Could you check a few things on this model? Use its own coordinates, in mm. Face numbers are marked on the shaded views. A direction names the side the tool comes from. Coordinates: 2 decimals unless noted, no trailing zeros. Loops run counter-clockwise (first coordinate to the right, second up) from the corner with the lowest first, then second, coordinate; pieces in that order, holes last.
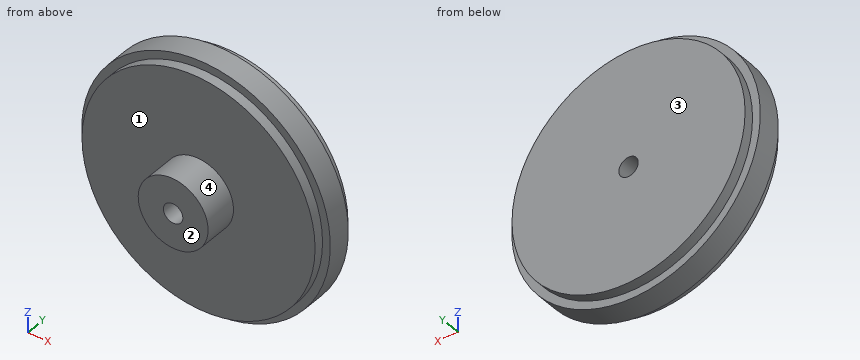
from build123d import *

# Parameters (mm, degrees)
SKETCH_1_R      = 32
SKETCH_1_R_2    = 30
EXTRUDE_1_DEPTH = 3
SKETCH_1_3_R    = 30
SKETCH_1_3_R_2  = 9
EXTRUDE_2_DEPTH = 5.5
SKETCH_1_5_R    = 9
SKETCH_1_5_R_2  = 2.5
EXTRUDE_3_DEPTH = 5.5
EXTRUDE_START   = -14
SKETCH_1_6_R    = 9
SKETCH_1_6_R_2  = 2.5
EXTRUDE_4_DEPTH = 14


with BuildPart() as part:
    # Sketch 1 → Extrude 1 (new, symmetric)
    with BuildSketch(Plane(origin=(0, 0, 0), x_dir=(1, 0, 0), z_dir=(0, 1, 0))):
        with Locations(Location((0, 0, 0), (0, 0, 270))):
            Circle(SKETCH_1_R)
        with Locations(Location((0, 0, 0), (0, 0, 270))):
            Circle(SKETCH_1_R_2, mode=Mode.SUBTRACT)
    extrude(amount=EXTRUDE_1_DEPTH, both=True)

    # Sketch 1_3 → Extrude 2 (add, symmetric)
    with BuildSketch(Plane(origin=(0, 0, 0), x_dir=(1, 0, 0), z_dir=(0, 1, 0))):
        with Locations(Location((0, 0, 0), (0, 0, 270))):
            Circle(SKETCH_1_3_R)
        with Locations(Location((0, 0, 0), (0, 0, 270))):
            Circle(SKETCH_1_3_R_2, mode=Mode.SUBTRACT)
    extrude(amount=EXTRUDE_2_DEPTH, both=True)

    # Sketch 1_5 → Extrude 3 (add)
    with BuildSketch(Plane(origin=(0, 0, 0), x_dir=(1, 0, 0), z_dir=(0, 1, 0))):
        with Locations(Location((0, 0, 0), (0, 0, 270))):
            Circle(SKETCH_1_5_R)
        with Locations(Location((0, 0, 0), (0, 0, 270))):
            Circle(SKETCH_1_5_R_2, mode=Mode.SUBTRACT)
    extrude(amount=EXTRUDE_3_DEPTH)

    # Sketch 1_6 → Extrude 4 (add)
    with BuildSketch(Plane(origin=(0, 0, 0), x_dir=(1, 0, 0), z_dir=(0, 1, 0)).offset(EXTRUDE_START)):
        with Locations(Location((0, 0, 0), (0, 0, 270))):
            Circle(SKETCH_1_6_R)
        with Locations(Location((0, 0, 0), (0, 0, 270))):
            Circle(SKETCH_1_6_R_2, mode=Mode.SUBTRACT)
    extrude(amount=EXTRUDE_4_DEPTH)


solid = part.part
(1) Imagine slicing it at B-B, the plane z = 0. Write out the boundary of the cut face in (x, y).
Answers:
outline: (-32, -3) - (-30, -3) - (-30, -5.5) - (-9, -5.5) - (-9, -14) - (-2.5, -14) - (-2.5, 5.5) - (-30, 5.5) - (-30, 3) - (-32, 3) - close; (2.5, -14) - (9, -14) - (9, -5.5) - (30, -5.5) - (30, -3) - (32, -3) - (32, 3) - (30, 3) - (30, 5.5) - (2.5, 5.5) - close
(2) For pin 1 (2 mm diameter, centred on y = -2.5, z = -20, fed in from -X); pin 2 (3 mm diameter, centred on y = 1, z = -4.5, fed in from +X); pin 3 (1.5 mm diameter, centred on x = 0.5, z = 2, fed in from +Y); pin 4 (5 mm diameter, centred on y = -9.5, z = -6.5, fed in from -X), each with a flat end and sliding along its axis, tell me the tip position at first contact or that it passes through.
Answers:
pin 1: stops at x = -25.75
pin 2: stops at x = 31.86
pin 3: stops at y = 5.5
pin 4: stops at x = -8.06
(3) Imagine slicing it at A-A, the plane x = 0. Write out the boundary of the cut face in (y, z), and give its area (4 significant figures).
Answers:
outline: (-14, -9) - (-5.5, -9) - (-5.5, -30) - (-3, -30) - (-3, -32) - (3, -32) - (3, -30) - (5.5, -30) - (5.5, -2.5) - (-14, -2.5) - close; (-14, 2.5) - (5.5, 2.5) - (5.5, 30) - (3, 30) - (3, 32) - (-3, 32) - (-3, 30) - (-5.5, 30) - (-5.5, 9) - (-14, 9) - close
area: 739.5 mm2
(4) Which directions (+Z, -Z, +X, -X, +Y, -Y) give clear straight access to the entire face, cutting with the end or side of a thin tool? Please do the marked faces 1 and 2.
Answers:
face 1: -Y
face 2: +Z, -Z, +X, -X, -Y
(5) Imagine slicing it at C-C, the plane y = -4.75. Write out the boundary of the cut face in (x, z), and give its area (3 significant figures).
Answers:
outline: circle Ø60 at (0, 0); hole circle Ø5 at (0, 0)
area: 2,810 mm2
(6) Imagine slicing it at D-D, the plane z = 16. Write out the boundary of the cut face in (x, y), and give its area (3 significant figures).
Answers:
outline: (-27.71, -3) - (-25.38, -3) - (-25.38, -5.5) - (25.38, -5.5) - (25.38, -3) - (27.71, -3) - (27.71, 3) - (25.38, 3) - (25.38, 5.5) - (-25.38, 5.5) - (-25.38, 3) - (-27.71, 3) - close
area: 586 mm2
(7) I need wall thicknesses on probe 1 along X at (y, z) = (-4.75, 0); probe 2 along X at (y, z) = (-0.5, 0); probe 3 along Y at (x, z) = (-23.5, -16.5). Which ranges of each line are inside material? Lowest first, please.
Answers:
probe 1: x = -30 to -2.5, 2.5 to 30
probe 2: x = -32 to -2.5, 2.5 to 32
probe 3: y = -5.5 to 5.5
(8) We'd pull the mould along X, two halves only. Please class the marked faces 3 and 4: +X half, -X half, draft (parallel to the pull), parting line (faces both ways), or undercut.
Answers:
face 3: draft
face 4: parting line
